For this review, take the finished solid that the model builds, in its own axes (mm). A direction names the side the tool comes from. Give positions to 0.01 mm unless a question says otherwise; leave off trailing zeros. Loops run counter-clockwise (first coordinate to the right, second up) from the corner with the lowest first, then second, coordinate; pieces in that order, holes last. Notation, with made-up numbers: M -37.75,68.5 L 8.25,68.5 A37 ccw 8.25,106.5 Z; hole C 74.25,-17 d2. An arc over 180 degrees is marked long. Use CSV: the item, a comma, the result in double quotes. Start each with the question number.
1. Tool access review of faces 1 (the face through (-52, 1.27, 74)), 2 (the face through (-43.157, 0, 72)), 3 (the face through (-54, 5, 2.458)), 4 (the face through (-52, -1.27, 74)), 5 (the face through (-60.937, 0, 72)): name each direction out of +Z, -Z, +X, -X, +Y, -Y from which nothing blocks a thin tool from reaching the whole face with its end or side.
2. The part is to be moulded in two halves that separate along Y. For faces 6 (the face through (-52, -7.62, 43)), 7 (the face through (-41.52, 5.33, 42.95)), 8 (the face through (-58.103, 1.907, 11.152)), say which applies: pulls with the +Y half, pulls with the -Y half, needs draft (parallel to the pull), parting line crosses it, or undercut.
3. Insertion check: P1, Ø1, axis at y = 2.5, z = 57.5, coming from the -X side; P2, Ø3, axis at y = -0.5, z = 74.5, coming from the +X side; P3, Ø2, axis at x = -47, z = 18, coming from the +Y side. Each pin has a flat end and moves straight along its axis. Give the tip position at first contact, or say it passes through.
4. Take a section at B-B, the plane y = -4. Write out the cut boundary in (x, z).
5. Take a section at D-D, the plane x = -63. Write out the cut boundary in (y, z).
6. To check wall thickness, follow line 1 (Z direction, x = -46.5, y = 2.25); line 2 (Z direction, x = -42.5, y = 1.5); line 3 (Y direction, x = -54.75, z = 74). State the ranges of each line that lie inside material, in increasing order. Write a range as [from, to].
7. Take a section at C-C, the plane x = -44.5. Write out the cut boundary in (y, z).
from build123d import *

# Parameters (mm, degrees)
F1_DEPTH = 7.62
F2_DEPTH = 1.27
F0_W     = 5.08
F0_H     = 42.841874063
F5_R     = 7.61999


# Not quite as in the source:
# - a fillet or chamfer is up to 0.001 mm smaller than in the source, because OpenCascade refuses the exact size


with BuildPart() as f1:
    # F0 (on Front) → F1 (new body, symmetric)
    with BuildSketch(Plane.XZ):
        Polygon((-45.6967013121, 20.0940572381), (-39.3467013121, 20.0940572381), (-39.3467013121, 65.1790572381), (-43.1567013121, 65.1790572381), (-60.9367013121, 65.1790572381), (-64.7467013121, 65.1790572381), (-64.7467013121, 20.0940572381), (-58.3967013121, 20.0940572381), (-52.0467013121, 20.0940572381), align=None)
    extrude(amount=F1_DEPTH, both=True)

    # F0 (on Front) → F2 (join, symmetric)
    with BuildSketch(Plane.XZ):
        with BuildLine():
            Line((-60.9367013121, 65.1790572381), (-43.1567013121, 65.1790572381))
            Line((-43.1567013121, 65.1790572381), (-43.1567013121, 79.1490572381))
            ThreePointArc((-43.1567013121, 79.1490572381), (-44.2726244757, 81.8431340744), (-46.9667013121, 82.9590572381))
            Line((-46.9667013121, 82.9590572381), (-57.1267013121, 82.9590572381))
            ThreePointArc((-57.1267013121, 82.9590572381), (-59.8207781484, 81.8431340744), (-60.9367013121, 79.1490572381))
            Line((-60.9367013121, 79.1490572381), (-60.9367013121, 65.1790572381))
        make_face()
    extrude(amount=F2_DEPTH, both=True)

    # F0 (on Front) → F3 (revolve)
    with BuildSketch(Plane.XZ):
        Polygon((-52.0467013121, 2.457652241), (-52.0467013121, 20.0940572381), (-58.3967013121, 20.0940572381), (-58.3967013121, 2.457652241), (-57.1267013121, 2.457652241), align=None)
    revolve(axis=Axis((-52.0467013121, 0, -10.145082292), (0, 0, -1)))

    # F0 (on Front) → F4 (revolve)
    with BuildSketch(Plane.XZ):
        with Locations((-54.5867013121, -18.9632847905)):
            Rectangle(F0_W, F0_H)
    revolve(axis=Axis((-52.0467013121, 0, -10.145082292), (0, 0, -1)))

    # F5 (radius 7.62 in the source; OpenCascade refuses exactly that, so slightly less here)
    f5_edges = [f1.edges().sort_by_distance(p)[0] for p in [
        (-39.346701, 7.62, 42.636557),
        (-64.746701, 7.62, 42.636557),
        (-64.746701, -7.62, 42.636557),
        (-39.346701, -7.62, 42.636557),
    ]]
    fillet(f5_edges, radius=F5_R)


solid = f1.part
Result set:
1,face 1,"+Z, +X, -X, +Y"
1,face 2,"+Z, +X, +Y, -Y"
1,face 3,"-Z"
1,face 4,"+Z, +X, -X, -Y"
1,face 5,"+Z, -X, +Y, -Y"
2,face 6,"pulls with the -Y half"
2,face 7,"pulls with the +Y half"
2,face 8,"parting line crosses it"
3,P1,"x = -64.48"
3,P2,"x = -43.16"
3,P3,"y = 4.89"
4,outline,"M -63.61,20.09 L -56.98,20.09 L -56.98,2.46 L -55.18,2.46 L -55.18,-40.38 L -48.92,-40.38 L -48.92,2.46 L -47.11,2.46 L -47.11,20.09 L -40.48,20.09 L -40.48,65.18 L -63.61,65.18 Z"
5,outline,"M -4.85,20.09 L 4.85,20.09 L 4.85,65.18 L -4.85,65.18 Z"
6,line 1,"[2.46, 65.18]"
6,line 2,"[20.09, 65.18]"
6,line 3,"[-1.27, 1.27]"
7,outline,"M -7.21,20.09 L 7.21,20.09 L 7.21,65.18 L 1.27,65.18 L 1.27,82.05 L -1.27,82.05 L -1.27,65.18 L -7.21,65.18 Z"
